Here's the drawing with two shaded views (mm, measured from the low corner). I have some questions. Give positions to 0.01 mm unless a question says otherwise; leave off trailing zeros. Loops run counter-clockwise (first coordinate to the right, second up) from the corner with the lowest first, then second, coordinate; pieces in that order, holes last. Notation, with made-up numbers: (-22, -40) -> (1, -40) arc R27 ccw to (1, -15) -> close; hole circle Ø4 at (84.25, 49.5). An arc over 180 degrees is marked (long way). Put each result on its own line as item: value.
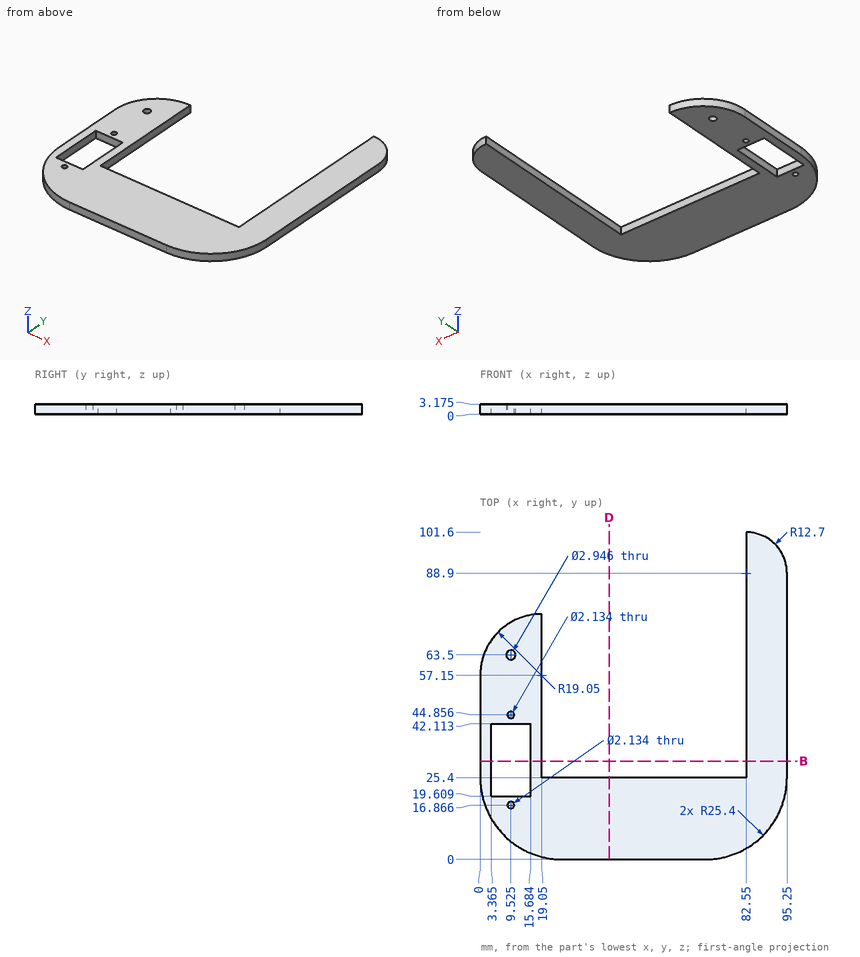
1. I'm going to push flat-ended pins straight in: pin 1 (1.5 mm diameter, centred on x = 27, z = 2.5, fed in from +Y); pin 2 (3.5 mm diameter, centred on x = 9.52, y = 44.86, fed in from +Z) (1 decimal). Where does each tip first touch, or does it pass through?
Recorded:
pin 1: stops at y = 25.4
pin 2: stops at z = 3.2
2. I need wall thicknesses on line 1 (X direction, y = 81.5, z = 1.8); line 2 (Y direction, x = 70.5, z = 0.85); line 3 (X direction, y = 16.5, z = 1.35). Which ranges of each line are inside material? Lowest first, please.
Recorded:
line 1: x = 82.55 to 95.25
line 2: y = 0.01 to 25.4
line 3: x = 1.61 to 8.52, 10.53 to 93.64
3. If we section it at B-B (y = 30.5): Count the separate pieces of the cut face and the enclosed holes in it.
Recorded:
separate pieces: 3
enclosed holes: 0
4. If we section it at D-D (x = 40): List the corners of the cut face in (y, z) for me (1 decimal).
Recorded:
outline: (0, 0) -> (25.4, 0) -> (25.4, 3.2) -> (0, 3.2) -> close
